from build123d import *

# Parameters (mm, degrees)
SKETCH1_R           = 1.5
BOSS_EXTRUDE1_DEPTH = 0.75


with BuildPart() as part:
    # Sketch1 → Boss-Extrude1 (new body, symmetric)
    with BuildSketch(Plane.XY):
        Polygon((-57.15, -23.8125), (57.15, -23.8125), (57.15, 23.8125), (50.8, 23.8125), (6.35, 4.7625), (-6.35, 4.7625), (-50.8, 23.8125), (-57.15, 23.8125), align=None)
        with Locations((53.975, 20.6375)):
            Circle(SKETCH1_R, mode=Mode.SUBTRACT)
        with Locations((53.975, 11.1125)):
            Circle(SKETCH1_R, mode=Mode.SUBTRACT)
        with Locations((-53.975, 20.6375)):
            Circle(SKETCH1_R, mode=Mode.SUBTRACT)
        with Locations((-53.975, 11.1125)):
            Circle(SKETCH1_R, mode=Mode.SUBTRACT)
    extrude(amount=BOSS_EXTRUDE1_DEPTH, both=True)


solid = part.part
Geometry check sheet. Reference: the model listing, model coordinates, mm. A direction names the side the tool comes from. Coordinates: 2 decimals unless noted, no trailing zeros. Order: outer loops, then holes, each group sorted by start corner. A loop starts at its lowest first (then second) coordinate and runs counter-clockwise, first axis right, second up. Notation, with made-up numbers: (31.25, 49) - (64.25, 49) arc R23 cw to (64.25, 58) - close; hole circle Ø9 at (61.5, 13). An arc over 180 degrees is marked (long way). One line per item, written item: value.
(1) Release check for a two-part mould opening along Y. For faces 3 (the face through (-28.264, 14.154, 0.01)), 4 (the face through (-1, -5, 0.75)), 5 (the face through (52.785, 10.2, -0.01)) record: +Y half, -Y half, draft (parallel to the pull), parting line (faces both ways), or undercut.
Data:
face 3: +Y half
face 4: draft
face 5: undercut
(2) Depth check by flat-ended pin: pin 1 Ø2.5 at (x, y) = (-53.98, 20.64) entering from -Z; pin 2 Ø0.8 at (x, z) = (-0.5, 0.5) entering from +Y. Enter the tip coordinate at first touch or a pass-through.
Data:
pin 1: passes through
pin 2: stops at y = 4.76
(3) Sectioned sample at C-C (x = 8). Enter the section's corners in (y, z), and give its area (3 significant figures).
Data:
outline: (-23.81, -0.75) - (5.47, -0.75) - (5.47, 0.75) - (-23.81, 0.75) - close
area: 43.9 mm^2
(4) Thickness scan on probe 1 along Y at (x, z) = (53, 0.4); probe 2 along X at (y, z) = (20, 0.15); probe 3 along X at (y, z) = (8.5, 0.1). Record the ranges inside material, lowest first. Write a range as from..to.
Data:
probe 1: y = -23.81..9.97, 12.25..19.5, 21.78..23.81
probe 2: x = -57.15..-55.33, -52.62..-41.9, 41.9..52.62, 55.33..57.15
probe 3: x = -57.15..-15.07, 15.07..57.15
(5) Sectioned sample at D-D (x = -9). Enter the section's corners in (y, z), and give its area (3 significant figures).
Data:
outline: (-23.81, -0.75) - (5.9, -0.75) - (5.9, 0.75) - (-23.81, 0.75) - close
area: 44.6 mm^2
(6) Access from +Z, -Z, +X, -X, +Y, -Y to the whole of each face (thin tool, end or side, straight path). Record for faces 1 (the face through (28.886, 14.421, 0.01)), 2 (the face through (52.87, 21.65, -0.01)).
Data:
face 1: +Z, -Z, +Y
face 2: +Z, -Z
(7) Sectioned sample at A-A (y = 16.5). Enter the section's corners in (x, z), and give its area (3 significant figures).
Data:
outline: (-57.15, -0.75) - (-33.74, -0.75) - (-33.74, 0.75) - (-57.15, 0.75) - close; (33.74, -0.75) - (57.15, -0.75) - (57.15, 0.75) - (33.74, 0.75) - close
area: 70.2 mm^2
(8) Sectioned sample at B-B (z = 0.1). Count the separate pieces of the cut face and the enclosed holes in it, and give its area (3 significant figures).
Data:
separate pieces: 1
enclosed holes: 4
area: 4,330 mm^2
